Can you work these out from the model? Positions are in its coordinate system, mm. Face numbers are marked on the shaded views. A direction names the side the tool comes from. Round coordinates to 2 decimals unless told otherwise and drop trailing zeros. Loops run counter-clockwise (first coordinate to the right, second up) from the corner with the lowest first, then second, coordinate; pieces in that order, holes last. Notation, with made-up numbers: (72, -24.5) -> (106, -24.5) arc R24 ccw to (106, 8.5) -> close; hole circle Ø8 at (25, 74). An arc over 180 degrees is marked (long way). Answer as a JSON object with one key per item and string values.
```python
from build123d import *

# Parameters (mm, degrees)
F1_DEPTH = 624.84
F3_W     = 222.237472
F3_H     = 523.24
F4_DEPTH = 99.06
F5_DEPTH = 627.38


with BuildPart() as f1:
    # F0 (on Front) → F1 (new body)
    with BuildSketch(Plane.XZ):
        with BuildLine():
            Line((363.537534, -301.646389), (401.637534, -301.646389))
            ThreePointArc((401.637534, -301.646389), (109.905185, -8.813365), (-182.561408, -300.913066))
            Line((-182.561408, -300.913066), (-144.461408, -300.913066))
            ThreePointArc((-144.461408, -300.913066), (109.905254, -46.913399), (363.537534, -301.646389))
        make_face()
    extrude(amount=F1_DEPTH)

    # F3 (on Top) → F4 (cut)
    with BuildSketch(Plane.XY):
        with Locations((102.249414, -312.42)):
            Rectangle(F3_W, F3_H)
    extrude(amount=-F4_DEPTH, mode=Mode.SUBTRACT)

    # F2 (on face) → F5 (join)
    with BuildSketch(Plane.XZ.offset(624.84)):
        with BuildLine():
            Line((176.094062, -55.787923), (222.495884, -249.826312))
            Line((222.495884, -249.826312), (0, -249.826312))
            Line((0, -249.826312), (-56.975495, -45.947485))
            ThreePointArc((-56.975495, -45.947485), (-91.072153, -3.893234), (-145.072013, 0))
            Line((-145.072013, 0), (-48.143223, -299.213022))
            Line((-48.143223, -299.213022), (310.081872, -299.213022))
            Line((310.081872, -299.213022), (251.000916, -45.353364))
            Line((251.000916, -45.353364), (176.094062, -55.787923))
        make_face()
    extrude(amount=-F5_DEPTH)


solid = f1.part
```
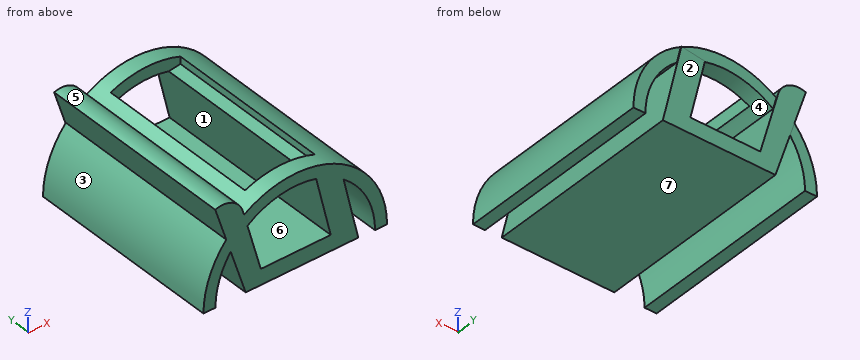
Q1. I want a section at A-A, the plane z = -193.5. Write out the boundary of the cut face in (x, y), then the cut area to 3 significant figures.
Determined:
{"outline": "(-162.1, -624.84) -> (-120.63, -624.84) -> (-120.63, 0) -> (-162.1, 0) -> close; (-82.39, -624.84) -> (-15.74, -624.84) -> (-15.74, 2.54) -> (-82.39, 2.54) -> close; (209.03, -624.84) -> (285.48, -624.84) -> (285.48, 2.54) -> (209.03, 2.54) -> close; (339.71, -624.84) -> (381.17, -624.84) -> (381.17, 0) -> (339.71, 0) -> close", "area": "142,000 mm²"}
Q2. I'm going to push flat-ended pins straight in: pin 1 (8 mm diameter, centred on x = 34.5, y = -157.5, fed in from -Z); pin 2 (10 mm diameter, centred on y = -107, z = -92.5, fed in from +X); pin 3 (19 mm diameter, centred on x = -167.5, y = -401.5, fed in from -Z). Where does each tip first touch, or does it pass through?
Determined:
{"pin 1": "z = -299.21", "pin 2": "x = 319.17", "pin 3": "z = -300.91"}
Q3. I want a section at D-D, the plane x = 288. Write out the boundary of the cut face in (y, z), then the cut area to 3 significant figures.
Determined:
{"outline": "(-624.84, -299.21) -> (2.54, -299.21) -> (2.54, -204.33) -> (-624.84, -204.33) -> close; (-624.84, -120.17) -> (0, -120.17) -> (0, -69.67) -> (-624.84, -69.67) -> close", "area": "91,100 mm²"}
Q4. On a 3-axis mill with a long thin cutter (end or side, diameter ignored), from which of +Z, -Z, +X, -X, +Y, -Y can I reach the whole of each face in a straight line? I mean the marked faces 5, 6 and 7. Say none if no direction works.
Determined:
{"face 5": "+Z, +Y, -Y", "face 6": "+Y, -Y", "face 7": "-Z, +Y, -Y"}
Q5. We'd pull the mould along X, two halves only. Please class the marked faces 1, 2, 3 and 4: pulls with the +X half, pulls with the -X half, needs draft (parallel to the pull), parting line crosses it, or undercut.
Determined:
{"face 1": "undercut", "face 2": "needs draft", "face 3": "pulls with the -X half", "face 4": "undercut"}
Q6. I want a section at C-C, the plane z = -84.5. Write out the boundary of the cut face in (x, y).
Determined:
{"outline": "(-117.7, -624.84) -> (-23.43, -624.84) -> (-23.43, 0) -> (-46.2, 0) -> (-46.2, 2.54) -> (-117.7, 2.54) -> close; (182.96, -624.84) -> (305.72, -624.84) -> (305.72, 0) -> (260.11, 0) -> (260.11, 2.54) -> (182.96, 2.54) -> close"}
Q7. I want a section at B-B, the plane x = 164.5. Write out the boundary of the cut face in (y, z), then the cut area to 3 significant figures.
Determined:
{"outline": "(-624.84, -299.21) -> (2.54, -299.21) -> (2.54, -249.83) -> (-624.84, -249.83) -> close; (-624.84, -52.93) -> (-574.04, -52.93) -> (-574.04, -14.03) -> (-624.84, -14.03) -> close; (-50.8, -52.93) -> (0, -52.93) -> (0, -14.03) -> (-50.8, -14.03) -> close", "area": "34,900 mm²"}
Q8. If I drill on L1, parallel to X at y = -531, z = -107.5; L2, parallel to X at y = -388, z = -176; L3, parallel to X at y = -94, z = -271, over which ranges is the centre line in solid material (lowest first)? Write a range as [from, to].
Determined:
{"L1": "[-110.25, -39.77], [188.46, 265.46], [274.18, 328.43]", "L2": "[-154.51, -111.62], [-88.06, -20.63], [204.84, 281.41], [330.7, 373.58]", "L3": "[-181.03, -142.69], [-57.28, 303.52], [361.77, 400.1]"}
